Source: CAD feature listing. Evaluate the final solid. Frame: model axes, mm. A direction names the side the tool comes from. Round coordinates to 2 decimals unless told otherwise and drop trailing zeros. Write each loop counter-clockwise with the first axis right and the second up, starting at its lowest first coordinate (ties: lowest second). Pieces come first, ordered by that corner, then holes. Notation, with made-up numbers: (2.5, 74) -> (43.5, 74) arc R19 ccw to (43.5, 89) -> close; hole circle Ø7 at (61, 38.25). An arc over 180 degrees is marked (long way). Put each result on its own line as item: value.
```python
from build123d import *

# Parameters (mm, degrees)
PAD_DEPTH       = 28
SKETCH001_R     = 19
POCKET_DEPTH    = 5
POCKET001_DEPTH = 26
SKETCH003_W     = 30
SKETCH003_H     = 6
POCKET002_DEPTH = 10
SKETCH004_W     = 2.8
SKETCH004_H     = 40
PAD001_DEPTH    = 5.8
SKETCH005_W     = 2.722469
SKETCH005_H     = 3
SKETCH005_W_2   = 2.715425
PAD002_DEPTH    = 12
SKETCH006_R     = 1.6
POCKET003_DEPTH = 5
SKETCH007_W     = 1
SKETCH007_H     = 4
POCKET004_DEPTH = 6
PAD003_DEPTH    = 10
SKETCH009_W     = 14.845783
SKETCH009_H     = 0.4
POCKET005_DEPTH = 0.4
SKETCH010_W     = 15.336478
SKETCH010_H     = 3
PAD004_DEPTH    = 32
SKETCH011_W     = 8.5
SKETCH011_H     = 24
POCKET006_DEPTH = 14
SKETCH012_W     = 0.8
SKETCH012_H     = 8.5
PAD005_DEPTH    = 24
SKETCH013_W     = 8.5
SKETCH013_H     = 0.4
POCKET007_DEPTH = 0.4


with BuildPart() as part:
    # Sketch → Pad (new body)
    with BuildSketch(Plane(origin=(0, 0, 0), x_dir=(1, 0, 0), z_dir=(0, 0, -1))):
        Polygon((-52.483848, 11.054775), (-10.483848, 11.054775), (-10.483848, 16.054775), (-24.483848, 32.054775), (-38.483848, 32.054775), (-52.483848, 16.054775), align=None)
    extrude(amount=PAD_DEPTH)

    # Sketch001 → Pocket (cut)
    with BuildSketch(Plane(origin=(0, -11.054775, 0), x_dir=(1, 0, 0), z_dir=(0, 1, 0))):
        with Locations((-31.483848, 21)):
            Circle(SKETCH001_R)
    extrude(amount=-POCKET_DEPTH, mode=Mode.SUBTRACT)

    # Sketch002 → Pocket001 (cut)
    with BuildSketch(Plane(origin=(0, 0, -28), x_dir=(1, 0, 0), z_dir=(0, 0, -1))):
        Polygon((-49.14737, 16.054775), (-36.483848, 32.054775), (-26.483848, 32.054775), (-13.820326, 16.054775), align=None)
    extrude(amount=-POCKET001_DEPTH, mode=Mode.SUBTRACT)

    # Sketch003 → Pocket002 (cut)
    with BuildSketch(Plane(origin=(0, 0, -28), x_dir=(1, 0, 0), z_dir=(0, 0, -1))):
        with Locations((-31.483848, 29.054775)):
            Rectangle(SKETCH003_W, SKETCH003_H)
    extrude(amount=-POCKET002_DEPTH, mode=Mode.SUBTRACT)

    # Sketch004 → Pad001 (new body)
    with BuildSketch(Plane(origin=(0, 0, -28), x_dir=(1, 0, 0), z_dir=(0, 0, -1))):
        with Locations((-46.98737, 40.454775)):
            Rectangle(SKETCH004_W, SKETCH004_H)
        with Locations((-15.98737, 40.454775)):
            Rectangle(SKETCH004_W, SKETCH004_H)
    extrude(amount=-PAD001_DEPTH)

    # Sketch005 → Pad002 (new body)
    with BuildSketch(Plane(origin=(0, 0, -28), x_dir=(1, 0, 0), z_dir=(0, 0, -1))):
        with Locations((-47.026135, 21.954775)):
            Rectangle(SKETCH005_W, SKETCH005_H)
        with Locations((-15.945082, 21.954775)):
            Rectangle(SKETCH005_W_2, SKETCH005_H)
    extrude(amount=-PAD002_DEPTH)

    # Sketch006 → Pocket003 (cut)
    with BuildSketch(Plane(origin=(0, -11.054775, 0), x_dir=(1, 0, 0), z_dir=(0, 1, 0))):
        with Locations((-47.483848, 4)):
            Circle(SKETCH006_R)
        with Locations((-15.483848, 4)):
            Circle(SKETCH006_R)
    extrude(amount=-POCKET003_DEPTH, mode=Mode.SUBTRACT)

    # Sketch007 → Pocket004 (cut)
    with BuildSketch(Plane(origin=(0, 0, -28), x_dir=(1, 0, 0), z_dir=(0, 0, -1))):
        with Locations((-46.98737, 55.054775)):
            Rectangle(SKETCH007_W, SKETCH007_H)
        with Locations((-15.98737, 55.054775)):
            Rectangle(SKETCH007_W, SKETCH007_H)
    extrude(amount=-POCKET004_DEPTH, mode=Mode.SUBTRACT)

    # Sketch008 → Pad003 (new body)
    with BuildSketch(Plane(origin=(0, 0, -18), x_dir=(1, 0, 0), z_dir=(0, 0, -1))):
        Polygon((-32.222141, 44.054382), (-31.422141, 44.054382), (-31.422141, 32.054775), (-24.483848, 32.054775), (-24.483848, 31.254775), (-38.483848, 31.254775), (-38.483848, 32.054775), (-32.222141, 32.054775), align=None)
    extrude(amount=PAD003_DEPTH)

    # Sketch009 → Pocket005 (cut)
    with BuildSketch(Plane(origin=(0, -31.254775, 0), x_dir=(1, 0, 0), z_dir=(0, 1, 0))):
        with Locations((-31.447088, 18.2)):
            Rectangle(SKETCH009_W, SKETCH009_H)
    extrude(amount=-POCKET005_DEPTH, mode=Mode.SUBTRACT)

    # Sketch010 → Pad004 (new body)
    with BuildSketch(Plane(origin=(0, 0, -28), x_dir=(1, 0, 0), z_dir=(0, 0, -1))):
        Polygon((-49.421348, 19.554775), (-66.483848, 19.554775), (-66.483848, 14.554775), (-64.483848, 14.554775), (-64.483848, 16.554775), (-52.046348, 16.554775), align=None)
        with Locations((-56.815609, 12.554775)):
            Rectangle(SKETCH010_W, SKETCH010_H)
    extrude(amount=-PAD004_DEPTH)

    # Sketch011 → Pocket006 (cut)
    with BuildSketch(Plane(origin=(-66.483848, 0, 0), x_dir=(0, 1, 0), z_dir=(-1, 0, 0))):
        with Locations((-15.304775, 12)):
            Rectangle(SKETCH011_W, SKETCH011_H)
    extrude(amount=-POCKET006_DEPTH, mode=Mode.SUBTRACT)

    # Sketch012 → Pad005 (new body)
    with BuildSketch(Plane.XY.offset(-24)):
        with Locations((-64.083848, -15.304775)):
            Rectangle(SKETCH012_W, SKETCH012_H)
    extrude(amount=PAD005_DEPTH)

    # Sketch013 → Pocket007 (cut)
    with BuildSketch(Plane(origin=(-64.483848, 0, 0), x_dir=(0, 1, 0), z_dir=(-1, 0, 0))):
        with Locations((-15.304775, 0.2)):
            Rectangle(SKETCH013_W, SKETCH013_H)
        with Locations((-15.304775, 23.8)):
            Rectangle(SKETCH013_W, SKETCH013_H)
    extrude(amount=-POCKET007_DEPTH, mode=Mode.SUBTRACT)


solid = part.part
```
Q1. Pin query (flat end, axial travel): pin 1 (5.5 mm diameter, centred on x = -31.5, y = -36, fed in from +Z); pin 2 (3 mm diameter, centred on x = -29, y = -29.5, fed in from -Z); pin 3 (3 mm diameter, centred on y = -38.5, z = -24, fed in from +X); pin 4 (5 mm diameter, centred on y = -37.5, z = -15, fed in from -X). Return the tip coordinate at first contact, or that it passes through.
Ans:
pin 1: stops at z = -18
pin 2: stops at z = -2
pin 3: stops at x = -14.59
pin 4: passes through
Q2. Cut plane D-D on z = -4. Give the number of separate pieces and of enclosed holes in the cut face, and give its area (3 significant figures).
Ans:
separate pieces: 5
enclosed holes: 0
area: 191 mm^2
Q3. Cut plane A-A on y = -34. Output: boundary loops of the cut face in (x, z).
Ans:
outline: (-48.39, -28) -> (-45.59, -28) -> (-45.59, -22.2) -> (-48.39, -22.2) -> close; (-32.22, -28) -> (-31.42, -28) -> (-31.42, -18) -> (-32.22, -18) -> close; (-17.39, -28) -> (-14.59, -28) -> (-14.59, -22.2) -> (-17.39, -22.2) -> close
Q4. Cut plane C-C on y = -51. Output: boundary loops of the cut face in (x, z).
Ans:
outline: (-48.39, -28) -> (-45.59, -28) -> (-45.59, -22.2) -> (-48.39, -22.2) -> close; (-17.39, -28) -> (-14.59, -28) -> (-14.59, -22.2) -> (-17.39, -22.2) -> close
Q5. Material intervals for line 1 (X direction, y = -14.9, z = -21); line 2 (X direction, y = -14, z = -4); line 3 (Z direction, x = -62, y = -18), sorted ascending. Write a range as [from, to].
Ans:
line 1: x = [-64.48, -63.68], [-52.48, -50.48], [-12.48, -10.48]
line 2: x = [-64.48, -63.68], [-52.48, -49.08], [-45.88, -39.97], [-23, -17.08], [-13.88, -10.48]
line 3: z = [-28, -24], [0, 4]
Q6. Cut plane B-B on x = -53.5. Output: boundary loops of the cut face in (y, z).
Ans:
outline: (-19.55, -28) -> (-16.55, -28) -> (-16.55, -24) -> (-19.55, -24) -> close; (-19.55, 0) -> (-16.55, 0) -> (-16.55, 4) -> (-19.55, 4) -> close; (-14.05, -28) -> (-11.05, -28) -> (-11.05, -24) -> (-14.05, -24) -> close; (-14.05, 0) -> (-11.05, 0) -> (-11.05, 4) -> (-14.05, 4) -> close
Q7. Draft query along Z for faces 1 (the flat face through (-48, -27, -28)), 2 (the flat face through (-31.422, -38, -23)), 3 (the cylindrical face through (-23.99, -13.52, -3.54)). Return one class per face: +Z half, -Z half, draft (parallel to the pull), parting line (faces both ways), or undercut.
Ans:
face 1: -Z half
face 2: draft
face 3: undercut
Q8. Reachability of faces 4 (the cylindrical face through (-13.958, -13.52, -4.481)), 5 (the flat face through (-47, -23.455, -19)), 6 (the flat face through (-48.387, -22, -19)), 7 (the flat face through (-50, -14.055, -21)), 8 (the flat face through (-46.487, -55, -25)) from +Z, -Z, +X, -X, +Y, -Y: full face, straight path, thin tool, end or side. Return the list, or none.
Ans:
face 4: +Y
face 5: +Z, -X, -Y
face 6: +Z, -Z, -X, -Y
face 7: none
face 8: +Z, -Z
